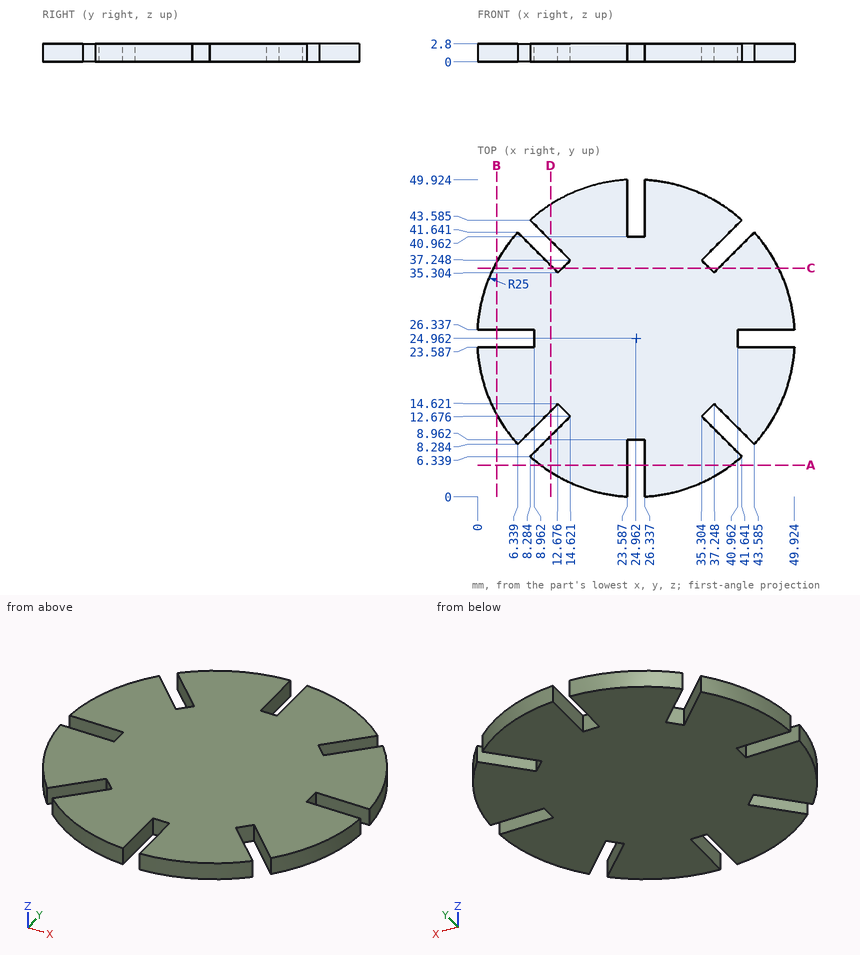
Answer from the drawing. Dimensions are ordinates in mm from the lowest x, y and z of the part. Coordinates: 2 decimals unless noted, no trailing zeros. Write each loop counter-clockwise with the first axis right and the second up, starting at its lowest first coordinate (ties: lowest second). Pieces come first, ordered by that corner, then holes. Notation, with made-up numbers: M -21.75,21.25 L 16.25,21.25 A32 ccw 16.25,49.25 Z; hole C 22,82 d9. An arc over 180 degrees is marked long. Write item = value, one per line.
1. Straight lines are drawn through the part: line 1 (X direction, y = 12, z = 1.65) (1 decimal); line 2 (X direction, y = 13, z = 0.6) (1 decimal); line 3 (Y direction, x = 26.5, z = 1.8) (1 decimal). For each, find the intervals that lie inside material, in ascending order. Write a range as from..to.
Solution:
line_1 = 3.6..10.1, 13.9..36, 39.9..46.3
line_2 = 3..11.1, 14.3..35.6, 38.9..46.9
line_3 = 0..49.9
2. The part is cut by section C-C (y = 36). Determine the outline of the cut face in (x, z) (1 decimal), then the cut area to 3 significant figures.
Solution:
outline = M 2.5,0 L 12,0 L 12,2.8 L 2.5,2.8 Z; M 13.4,0 L 36.6,0 L 36.6,2.8 L 13.4,2.8 Z; M 37.9,0 L 47.4,0 L 47.4,2.8 L 37.9,2.8 Z
area = 118 mm2
3. The part is cut by section D-D (x = 11.5). Determine the outline of the cut face in (y, z) (1 decimal).
Solution:
outline = M 3.9,0 L 9.6,0 L 9.6,2.8 L 3.9,2.8 Z; M 13.4,0 L 36.5,0 L 36.5,2.8 L 13.4,2.8 Z; M 40.4,0 L 46,0 L 46,2.8 L 40.4,2.8 Z
4. Flat-ended cylindrical pins translate along their axes: pin 1 (1.5 mm diameter, centred on x = 25.5, z = 1, fed in from -Y); pin 2 (1.4 mm diameter, centred on x = 3, z = 1, fed in from +Y); pin 3 (1.4 mm diameter, centred on y = 25, z = 1.5, fed in from -X). Find the tip coordinate at first contact, or state that the pin passes through.
Solution:
pin_1 = 8.96
pin_2 = 38.11
pin_3 = 8.96
5. The part is cut by section B-B (x = 3). Determine the outline of the cut face in (y, z).
Solution:
outline = M 13.02,0 L 23.59,0 L 23.59,2.8 L 13.02,2.8 Z; M 26.34,0 L 36.91,0 L 36.91,2.8 L 26.34,2.8 Z
6. The part is cut by section A-A (y = 5). Determine the outline of the cut face in (x, z).
Solution:
outline = M 9.91,0 L 23.59,0 L 23.59,2.8 L 9.91,2.8 Z; M 26.34,0 L 40.01,0 L 40.01,2.8 L 26.34,2.8 Z
